Can you work these out from the model? Positions are in its coordinate system, mm. A direction names the side the tool comes from. Give positions to 0.01 mm unless a question says otherwise; leave off trailing zeros. Write each loop counter-clockwise with the first axis right and the second up, starting at its lowest first coordinate (ties: lowest second). Pieces come first, ordered by that corner, then holes.
```python
from build123d import *

# Parameters (mm, degrees)
BOSS_EXTRUDE1_DEPTH = 5


with BuildPart() as part:
    # Sketch2 → Boss-Extrude1 (new body)
    with BuildSketch(Plane.XY):
        with BuildLine():
            Line((3.000022, 125.605083), (0, 125.605083))
            Line((0, 125.605083), (0, 131.876887))
            Line((0, 131.876887), (8.190395777, 131.876887))
            Line((8.190395777, 131.876887), (8.190395777, 128.876921))
            Line((8.190395777, 128.876921), (16.281283777, 128.876921))
            Line((16.281283777, 128.876921), (16.281283777, 131.876908))
            Line((16.281283777, 131.876908), (24.572181777, 131.876908))
            Line((24.572181777, 131.876908), (24.572181777, 128.876921))
            Line((24.572181777, 128.876921), (32.663126777, 128.876921))
            Line((32.663126777, 128.876921), (32.663126777, 131.876908))
            Line((32.663126777, 131.876908), (40.954024777, 131.876908))
            Line((40.954024777, 131.876908), (40.954024777, 128.876921))
            Line((40.954024777, 128.876921), (49.032014777, 128.876921))
            Line((49.032014777, 128.876921), (49.032014777, 131.870876))
            Line((49.032014777, 131.870876), (78.034171777, 131.870876))
            add(Edge.make_bspline(
                [(78.034171777, 131.870876), (79.118469777, 131.870876), (79.997507777, 130.991859), (79.998212777, 129.914053)],
                knots=[0, 0, 0, 0, 1, 1, 1, 1], degree=3))
            Line((79.998212777, 129.914053), (80.048932, 0.769332))
            add(Edge.make_bspline(
                [(78.08681, -1.164385), (79.171108, -1.164385), (80.050118, -0.285367), (80.048932, 0.769332)],
                knots=[0, 0, 0, 0, 1, 1, 1, 1], degree=3))
            Line((78.08681, -1.164385), (57.273444, -1.164385))
            Line((57.273444, -1.164385), (57.273444, 1.835025))
            Line((57.273444, 1.835025), (49.182528, 1.835025))
            Line((49.182528, 1.835025), (49.182528, -1.165))
            Line((49.182528, -1.165), (40.904555, -1.165))
            Line((40.904555, -1.165), (40.904555, 1.835025))
            Line((40.904555, 1.835025), (32.813639, 1.835025))
            Line((32.813639, 1.835025), (32.813639, -1.165))
            Line((32.813639, -1.165), (24.522769, -1.165))
            Line((24.522769, -1.165), (24.522769, 1.835025))
            Line((24.522769, 1.835025), (16.431825, 1.835025))
            Line((16.431825, 1.835025), (16.431825, -1.164385))
            Line((16.431825, -1.164385), (8.140926, -1.164385))
            Line((8.140926, -1.164385), (8.140926, 1.835025))
            Line((8.140926, 1.835025), (0.026314406, 1.835025))
            Line((0.026314406, 1.835025), (0.026314406, 8.841283))
            Line((0.026314406, 8.841283), (3.000022, 8.841283))
            Line((3.000022, 8.841283), (3.000022, 16.532191))
            Line((3.000022, 16.532191), (0.026314406, 16.532191))
            Line((0.026314406, 16.532191), (0.026314406, 24.423125))
            Line((0.026314406, 24.423125), (3.000022, 24.423125))
            Line((3.000022, 24.423125), (3.000022, 32.114033))
            Line((3.000022, 32.114033), (0, 32.114033))
            Line((0, 32.114033), (0, 40.004966))
            Line((0, 40.004966), (3.000022, 40.004966))
            Line((3.000022, 40.004966), (3.000022, 47.695875))
            Line((3.000022, 47.695875), (0, 47.695875))
            Line((0, 47.695875), (0, 55.586808))
            Line((0, 55.586808), (3.000022, 55.586808))
            Line((3.000022, 55.586808), (3.000022, 63.277716))
            Line((3.000022, 63.277716), (0, 63.277716))
            Line((0, 63.277716), (0, 71.16865))
            Line((0, 71.16865), (3.000022, 71.16865))
            Line((3.000022, 71.16865), (3.000022, 78.859558))
            Line((3.000022, 78.859558), (0, 78.859558))
            Line((0, 78.859558), (0, 86.750491))
            Line((0, 86.750491), (3.000022, 86.750491))
            Line((3.000022, 86.750491), (3.000022, 94.4414))
            Line((3.000022, 94.4414), (0, 94.4414))
            Line((0, 94.4414), (0, 102.332333))
            Line((0, 102.332333), (3.000022, 102.332333))
            Line((3.000022, 102.332333), (3.000022, 110.023241))
            Line((3.000022, 110.023241), (0, 110.023241))
            Line((0, 110.023241), (0, 117.914175))
            Line((0, 117.914175), (3.000022, 117.914175))
            Line((3.000022, 117.914175), (3.000022, 125.605083))
        make_face()
        with BuildLine():
            add(Edge.make_bspline(
                [(58.942475583, 4.45705786), (58.876355433, 3.116936717), (59.910031097, 1.976908278), (61.249001885, 1.910844885)],
                knots=[0, 0, 0, 0, 1, 1, 1, 1], degree=3))
            add(Edge.make_bspline(
                [(61.249001885, 1.910844885), (62.61708533, 1.904036469), (63.733535737, 3.008514398), (63.740350017, 4.377776229)],
                knots=[0, 0, 0, 0, 1, 1, 1, 1], degree=3))
            add(Edge.make_bspline(
                [(63.740350017, 4.377776229), (63.747057434, 5.712148161), (62.669459301, 6.79974011), (61.335720144, 6.806444347)],
                knots=[0, 0, 0, 0, 1, 1, 1, 1], degree=3))
            add(Edge.make_bspline(
                [(61.335720144, 6.806444347), (60.026995423, 6.818478401), (58.95451532, 5.766400599), (58.942475583, 4.45705786)],
                knots=[0, 0, 0, 0, 1, 1, 1, 1], degree=3))
        make_face(mode=Mode.SUBTRACT)
        with BuildLine():
            add(Edge.make_bspline(
                [(58.81372287, 126.294450328), (58.82088208, 124.91026836), (59.949710178, 123.793975081), (61.332703971, 123.801128146)],
                knots=[0, 0, 0, 0, 1, 1, 1, 1], degree=3))
            add(Edge.make_bspline(
                [(61.332703971, 123.801128146), (62.683823094, 123.814309965), (63.770278691, 124.921256436), (63.757085518, 126.273539334)],
                knots=[0, 0, 0, 0, 1, 1, 1, 1], degree=3))
            add(Edge.make_bspline(
                [(63.757085518, 126.273539334), (63.749960977, 127.651200571), (62.626009819, 128.762672593), (61.249001885, 128.755551431)],
                knots=[0, 0, 0, 0, 1, 1, 1, 1], degree=3))
            add(Edge.make_bspline(
                [(61.249001885, 128.755551431), (59.897851275, 128.748355096), (58.806523136, 127.646238991), (58.81372287, 126.294450328)],
                knots=[0, 0, 0, 0, 1, 1, 1, 1], degree=3))
        make_face(mode=Mode.SUBTRACT)
    extrude(amount=BOSS_EXTRUDE1_DEPTH)


solid = part.part
```
1) For faces 1 (the face through (16.432, 0, 2)), 2 (the face through (3, 59, 2)), 3 (the face through (8.19, 130, 2)), which set-ups out of +Z, -Z, +X, -X, +Y, -Y let a thin tool reach every point of the face, with its end or its side?
Values follow:
face 1: +Z, -Z, -Y
face 2: +Z, -Z, -X
face 3: +Z, -Z, +Y
2) Suppose I cut it at A-A on x = 19. Write out the boundary of the cut face in (y, z), plus the area to 3 significant figures.
Values follow:
outline: (1.84, 0) - (131.88, 0) - (131.88, 5) - (1.84, 5) - close
area: 650 mm2
3) For pin 1 Ø1.5 at (x, z) = (1, 3) entering from -Y (3 decimals); pin 2 Ø1.5 at (y, z) = (34, 3.5) entering from +X; pin 3 Ø1 at (x, z) = (28.5, 1.5) entering from +Y, each with a flat end and sliding along its axis, tell me the tip position at first contact or that it passes through.
Values follow:
pin 1: stops at y = 1.835
pin 2: stops at x = 80.04
pin 3: stops at y = 128.88
4) Suppose I cut it at B-B on z = 3.65. State how many separate pieces and enclosed holes the cut face has, plus the area to 3 significant figures.
Values follow:
separate pieces: 1
enclosed holes: 2
area: 10,300 mm2
5) Suppose I cut it at C-C on y = 42.5. Write out the boundary of the cut face in (x, z).
Values follow:
outline: (3, 0) - (80.03, 0) - (80.03, 5) - (3, 5) - close
6) Please list where these lines run through material, in increasing order: L1, parallel to X at y = 13, z = 3.6; L2, parallel to X at y = 48.5, z = 1.85; L3, parallel to Y at x = 34, z = 0.9.
Values follow:
L1: x = 3 to 80.04
L2: x = 0 to 80.03
L3: y = 1.84 to 131.88
7) If we mould it in two halves opening along Y, with no side actions, what happens to faces 4 (the face through (8.141, 0, 2)), 5 (the face through (3, 75, 2)), 6 (the face through (2, 47.696, 2)), 7 (the face through (12, 128.877, 2))? For each: +Y half, -Y half, draft (parallel to the pull), parting line (faces both ways), or undercut.
Values follow:
face 4: draft
face 5: undercut
face 6: undercut
face 7: +Y half
